Check sheet for the modelled part. Datum: model origin and axes. Units: mm. A direction names the side the tool comes from. Round coordinates to 2 decimals unless told otherwise and drop trailing zeros. Write each loop counter-clockwise with the first axis right and the second up, starting at its lowest first coordinate (ties: lowest second). Pieces come first, ordered by that corner, then holes.
Item 1: Cross-section at B-B on x = 0. Enter the section's corners in (y, z).
Item 2: Cross-section at A-A on z = 0.3. Enter the section's corners in (x, y).
Item 3: Release check for a two-part mould opening along Y. For faces 4 (the flat face through (0, 0, 1.7)), 5 (the flat face through (0, 6.5, 1)), 6 (the flat face through (4, 0, 2)), 7 (the cylindrical face through (-0.54, 2.44, 3.99)) record: +Y half, -Y half, draft (parallel to the pull), parting line (faces both ways), or undercut.
Item 4: Cross-section at C-C on y = 0. Enter the section's corners in (x, z), plus the area to 3 significant figures.
Item 5: Material ranges on line 1 (Y direction, x = 0, z = 4.3); line 2 (X direction, y = 2, z = 1.4); line 3 (Y direction, x = -0.5, z = 1.2), recorded low to high.
Item 6: Cross-section at D-D on y = 2.75. Enter the section's corners in (x, z).
Item 7: Go/stop test with flat-tipped pins: pin 1 Ø2.5 at (x, y) = (0, 0) entering from +Z; pin 2 Ø1.5 at (x, y) = (0.5, 1.5) entering from -Z. Record where each tip stops, or that it passes through.
Item 8: Tool access check on faces 1 (the cylindrical face through (-1.5, -0.07, 3.99)), 2 (the flat face through (0, -6.5, 1)), 3 (the flat face through (-3, 0, 0)). Record the directions out of +Z, -Z, +X, -X, +Y, -Y that give a thin tool (end or side, any length) a straight path to the whole face; none if there is none.
Autodesk Inventor part; units mm, degrees
ref_plane "YZ Plane" through (0, 0, 0) normal (1, 0, 0) x (0, 1, 0)
ref_plane "XZ Plane" through (0, 0, 0) normal (0, 1, 0) x (-1, 0, 0)
ref_plane "XY Plane" through (0, 0, 0) normal (0, 0, 1) x (1, 0, 0)
sketch "Sketch1" plane through (0, 0, 0) normal (0, 0, 1) x (1, 0, 0)
  line L0 (-4, 8) -> (4, 8)
  line L1 (4, 8) -> (4, -8)
  line L2 (4, -8) -> (-4, -8)
  line L3 (-4, -8) -> (-4, 8)
  point P0 (0, 0)
  dimension "d0" = 8
  dimension "d1" = 16
  dimension "d2" = 4
  dimension "d3" = 8
extrude "Extrusion1" add sketch "Sketch1" along normal blind 3.2
shell "Shell1" thickness 1.5 removed faces 1 at (-1.3333, 2.6667, 0)
sketch "Sketch2" plane through (0, 0, 3.2) normal (0, 0, 1) x (1, 0, 0)
  circle A0 centre (0, -4) radius 2.5
  line L0 (4, 8) -> (4, -8)
  line L1 (4, -8) -> (-4, -8)
  dimension "d7" = 5
  dimension "d10" = 4
  dimension "d11" = 4
extrude "Extrusion2" [suppressed]
sketch "Sketch3" plane through (2.5, -6.5, 1.7) normal (0, 0, -1) x (-1, 0, 0)
  point P0 (2.5, 6.5)
extrude "Extrusion3" [suppressed]
pattern_linear "Rectangular Pattern1" [suppressed]
sketch "Sketch4" plane through (2.5, -6.5, 1.7) normal (0, 0, -1) x (-1, 0, 0)
  point P0 (2.5, 6.5)
extrude "Extrusion4" [suppressed]
pattern_linear "Rectangular Pattern2" [suppressed]
sketch "Sketch5" plane through (0, 0, 3.2) normal (0, 0, 1) x (1, 0, 0)
  circle A0 centre (0, 0) radius 2.5
  circle A1 centre (0, 0) radius 1.5
  dimension "d41" = 5
  dimension "d42" = 3
extrude "Extrusion5" add sketch "Sketch5" along normal blind 1.6
equation "\"d0\" = 0.8 * WIDTH"
equation "\"d1\" = 0.8 * LENGTH"
equation "\"d4\" = HEIGHT"
equation "\"WIDTH\" = 1"
equation "\"HEIGHT\" = 3.2"
properties part number "3794" material "Steel"
Response values:
1. outline: (-8, 0) - (-6.5, 0) - (-6.5, 1.7) - (6.5, 1.7) - (6.5, 0) - (8, 0) - (8, 3.2) - (2.5, 3.2) - (2.5, 4.8) - (1.5, 4.8) - (1.5, 3.2) - (-1.5, 3.2) - (-1.5, 4.8) - (-2.5, 4.8) - (-2.5, 3.2) - (-8, 3.2) - close
2. outline: (-4, -8) - (4, -8) - (4, 8) - (-4, 8) - close; hole (-2.5, -6.5) - (2.5, -6.5) - (2.5, 6.5) - (-2.5, 6.5) - close
3. face 4: undercut
3. face 5: undercut
3. face 6: draft
3. face 7: parting line
4. outline: (-4, 0) - (-2.5, 0) - (-2.5, 1.7) - (2.5, 1.7) - (2.5, 0) - (4, 0) - (4, 3.2) - (2.5, 3.2) - (2.5, 4.8) - (1.5, 4.8) - (1.5, 3.2) - (-1.5, 3.2) - (-1.5, 4.8) - (-2.5, 4.8) - (-2.5, 3.2) - (-4, 3.2) - close
4. area: 20.3 mm2
5. line 1: y = -2.5 to -1.5, 1.5 to 2.5
5. line 2: x = -4 to -2.5, 2.5 to 4
5. line 3: y = -8 to -6.5, 6.5 to 8
6. outline: (-4, 0) - (-2.5, 0) - (-2.5, 1.7) - (2.5, 1.7) - (2.5, 0) - (4, 0) - (4, 3.2) - (-4, 3.2) - close
7. pin 1: stops at z = 3.2
7. pin 2: stops at z = 1.7
8. face 1: +Z
8. face 2: -Z
8. face 3: -Z, +X, -X, +Y, -Y
